Verification items for this drawing (mm, ordinates from the low corner). A direction names the side the tool comes from. Round coordinates to 2 decimals unless told otherwise and drop trailing zeros. Order: outer loops, then holes, each group sorted by start corner. A loop starts at its lowest first (then second) coordinate and runs counter-clockwise, first axis right, second up.
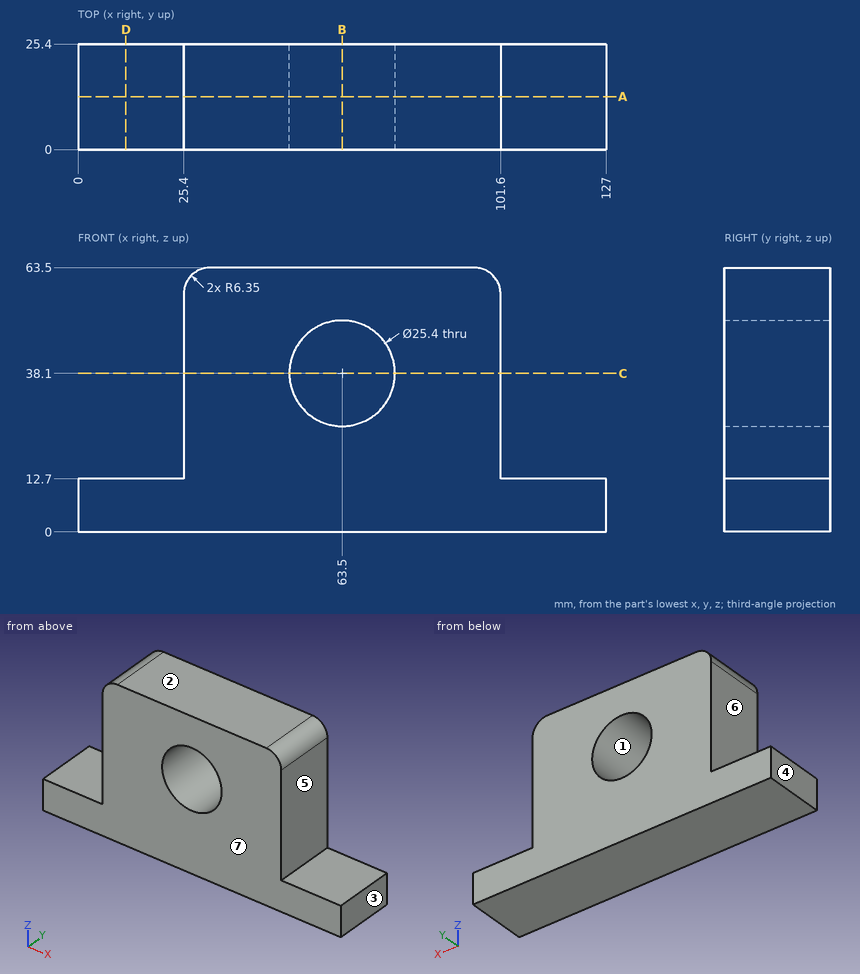
Item 1: Go/stop test with flat-tipped pins: P1, Ø12, axis at y = 15, z = 51, coming from the -X side; P2, Ø2, axis at x = 104.5, y = 12.5, coming from the +Z side; P3, Ø12.5, axis at y = 18, z = 41.5, coming from the +X side; P4, Ø23, axis at x = 63.5, z = 38.1, coming from the -Y side. Record where each tip stops, or that it passes through.
Answer:
P1: stops at x = 25.4
P2: stops at z = 12.7
P3: stops at x = 101.6
P4: passes through
Item 2: Sectioned sample at A-A (y = 12.75). Record the cut outline in (x, z).
Answer:
outline: (0, 0) - (127, 0) - (127, 12.7) - (101.6, 12.7) - (101.6, 57.15) arc R6.35 ccw to (95.25, 63.5) - (31.75, 63.5) arc R6.35 ccw to (25.4, 57.15) - (25.4, 12.7) - (0, 12.7) - close; hole circle Ø25.4 at (63.5, 38.1)
Item 3: Sectioned sample at C-C (z = 38.1). Record the cut outline in (x, y), and give its area (3 significant figures).
Answer:
outline: (25.4, 0) - (50.8, 0) - (50.8, 25.4) - (25.4, 25.4) - close; (76.2, 0) - (101.6, 0) - (101.6, 25.4) - (76.2, 25.4) - close
area: 1,290 mm2
Item 4: Sectioned sample at D-D (x = 11.5). Record the cut outline in (y, z).
Answer:
outline: (0, 0) - (25.4, 0) - (25.4, 12.7) - (0, 12.7) - close
Item 5: Scan lines: line 1 along Z through (x, y) = (63.5, 5.5); line 2 along Z through (x, y) = (31.5, 4.5); line 3 along X through (y, z) = (14.25, 43). Record each from-to range of solid material in increasing order.
Answer:
line 1: z = 0 to 25.4, 50.8 to 63.5
line 2: z = 0 to 63.5
line 3: x = 25.4 to 51.78, 75.22 to 101.6
Item 6: Sectioned sample at B-B (x = 63.5). Record the cut outline in (y, z), and give its area (3 significant figures).
Answer:
outline: (0, 0) - (25.4, 0) - (25.4, 25.4) - (0, 25.4) - close; (0, 50.8) - (25.4, 50.8) - (25.4, 63.5) - (0, 63.5) - close
area: 968 mm2
Item 7: Release check for a two-part mould opening along X. For the marked faces 1, 2, 3 and 4 record: released by +X, released by -X, zero draft, split by the parting line, or undercut.
Answer:
face 1: undercut
face 2: zero draft
face 3: released by +X
face 4: released by -X
Item 8: Access from +Z, -Z, +X, -X, +Y, -Y to the whole of each face (thin tool, end or side, straight path). Record for the marked faces 5, 6 and 7.
Answer:
face 5: +Z, +X, +Y, -Y
face 6: +Z, -X, +Y, -Y
face 7: +Z, -Z, +X, -X, -Y
